The figure shows three views and two pictorial views of one solid part (mm, origin at its lowest corner). Answer the questions. A direction names the side the tool comes from. Give positions to 0.01 mm unless a question says otherwise; leave off trailing zeros. Loops run counter-clockwise (first coordinate to the right, second up) from the corner with the lowest first, then second, coordinate; pieces in that order, holes last. Notation, with made-up numbers: (34, -25.5) - (75, -25.5) arc R15 ccw to (75, -7.5) - close; hole circle Ø11 at (46.25, -22). An arc over 180 degrees is marked (long way). Use a Markdown table: item, result. Add a question column.
Item 1: A cutting plane is placed at D-D (x = 11). Determine the outline of the cut face in (y, z) (1 decimal), plus the area to 3 significant figures.
Item 2: A cutting plane is placed at A-A (x = 19.05). Determine the outline of the cut face in (y, z) (1 decimal).
Item 3: A cutting plane is placed at B-B (z = 49). Determine the outline of the cut face in (x, y) (1 decimal), plus the area to 3 significant figures.
Item 4: Each of these flat-tipped pins is pushed along its axis until it touches: P1, Ø11.5, axis at x = 8.255, y = 12.446, coming from the +Z side; P2, Ø5, axis at x = 29.5, z = 18.5, coming from the -Y side (3 decimals); P3, Ø5, axis at x = 7.5, z = 34, coming from the -Y side; P4, Ø14, axis at x = 21, y = 15.5, coming from the -Z side. Where does it stop, or does it pass through?
Item 5: Which of the six approach directions +Z, -Z, +X, -X, +Y, -Y give full straight-line access (tool end or side, diameter ignored) to the marked faces 1, 2 and 3?
Item 6: A cutting plane is placed at C-C (y = 15.25). Determine the outline of the cut face in (x, z) (1 decimal), plus the area to 3 significant figures.
Item 7: Consider probe 1 along Z at (x, y) = (17, 17.75) (1 decimal); probe 2 along Y at (x, z) = (3, 26.5) (1 decimal); probe 3 along Y at (x, z) = (3, 38) (1 decimal). Determine where each line is inside the solid, lowest interval first. Write a range as [from, to].
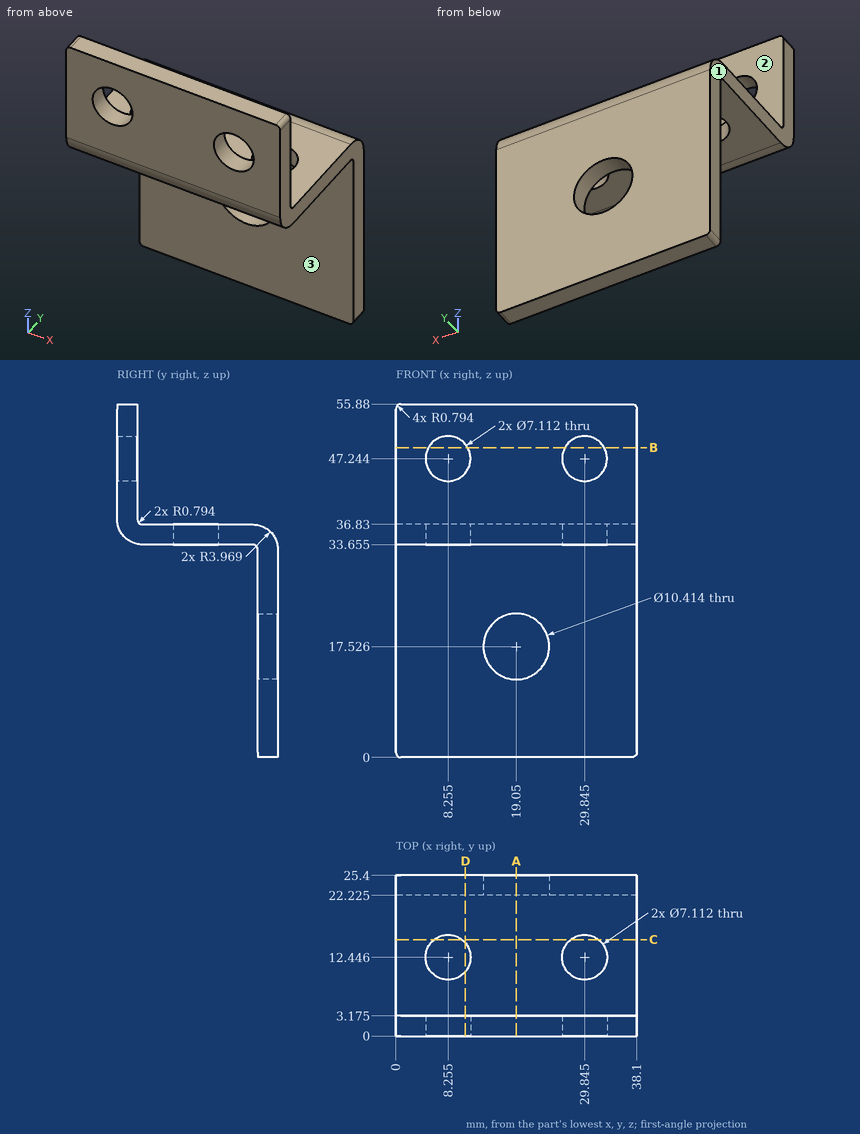
Geometry says:
| question | item | result |
|---|---|---|
| 1 | outline | (0, 37.6) arc R4 ccw to (4, 33.7) - (10.2, 33.7) - (10.2, 36.8) - (4, 36.8) arc R0.8 cw to (3.2, 37.6) - (3.2, 45) - (0, 45) - close; (0, 49.5) - (3.2, 49.5) - (3.2, 55.9) - (0, 55.9) - close; (14.7, 33.7) - (21.4, 33.7) arc R0.8 cw to (22.2, 32.9) - (22.2, 0) - (25.4, 0) - (25.4, 32.9) arc R4 ccw to (21.4, 36.8) - (14.7, 36.8) - close |
| 1 | area | 213 mm² |
| 2 | outline | (0, 37.6) arc R4 ccw to (4, 33.7) - (21.4, 33.7) arc R0.8 cw to (22.2, 32.9) - (22.2, 22.7) - (25.4, 22.7) - (25.4, 32.9) arc R4 ccw to (21.4, 36.8) - (4, 36.8) arc R0.8 cw to (3.2, 37.6) - (3.2, 55.9) - (0, 55.9) - close; (22.2, 0) - (25.4, 0) - (25.4, 12.3) - (22.2, 12.3) - close |
| 3 | outline | (0, 0) - (5.2, 0) - (5.2, 3.2) - (0, 3.2) - close; (11.3, 0) - (26.8, 0) - (26.8, 3.2) - (11.3, 3.2) - close; (32.9, 0) - (38.1, 0) - (38.1, 3.2) - (32.9, 3.2) - close |
| 3 | area | 81.7 mm² |
| 4 | P1 | z = 36.83 |
| 4 | P2 | y = 22.225 |
| 4 | P3 | y = 0.16 |
| 4 | P4 | z = 0 |
| 5 | face 1 | +Z, -Z, -X, +Y, -Y |
| 5 | face 2 | +Z, +X, -X, +Y |
| 5 | face 3 | -Z, +X, -X, -Y |
| 6 | outline | (0, 33.7) - (6.1, 33.7) - (6.1, 36.8) - (0, 36.8) - close; (10.4, 33.7) - (27.7, 33.7) - (27.7, 36.8) - (10.4, 36.8) - close; (32, 33.7) - (38.1, 33.7) - (38.1, 36.8) - (32, 36.8) - close |
| 6 | area | 93.2 mm² |
| 7 | probe 1 | [33.7, 36.8] |
| 7 | probe 2 | [22.2, 25.4] |
| 7 | probe 3 | [0, 3.2] |
